Geometry: final body of the model. Coordinates: model frame, mm. A direction names the side the tool comes from. Give positions to 0.01 mm unless a question says otherwise; leave off trailing zeros. Write each loop counter-clockwise with the first axis right and the second up, starting at its lowest first coordinate (ties: lowest second). Pieces come first, ordered by that corner, then holes. Notation, with made-up numbers: M 69.5,69.25 L 115.5,69.25 A15 ccw 115.5,91.25 Z; hole C -29,79.5 d1. An arc over 180 degrees is marked long. Use one line per item in the form item = value. Start each with the question number.
Item 1: Section query C-C on x = 7.75. Return loops of the section in (y, z), then the cut area to 3 significant figures.
Item 2: Material intervals for line 1 along X through (y, z) = (13.5, 200.5); line 2 along Y through (x, z) = (1, 281.5); line 3 along X through (y, z) = (15, 165), sorted ascending. Write a range as from..to.
Item 3: Section query A-A on y = -8. Return loops of the section in (x, z), then the cut area to 3 significant figures.
Item 4: Contact query for a flat-ended pin moving along its axis: P1, Ø3, axis at x = 0.53, z = 190.5, coming from the -Y side. Output: stop coordinate, or through.
Item 5: Pull-direction query (Y, two-part tool) for faces 3 (the flat face through (1, 14.737, 150)), 4 (the flat face through (13.229, -9, 150)), 5 (the flat face through (1, -34.793, 150)); classes: released by +Y, released by -Y, zero draft, split by the parting line, or undercut.
Item 6: Access query for faces 1 (the flat face through (-10.901, -9, 150)), 2 (the flat face through (-12.171, -10, 150)). Directions: +Z, -Z, +X, -X, +Y, -Y. A direction counts if a zero-diameter tool reaches every point of the face in a straight line with its end or side. Return the directions, or none.
Item 7: Section query B-B on z = 108. Return loops of the section in (x, y), then the cut area to 3 significant figures.
Autodesk Inventor part; units mm, degrees
ref_plane "YZ Plane" through (0, 0, 0) normal (1, 0, 0) x (0, 1, 0)
ref_plane "XZ Plane" through (0, 0, 0) normal (0, 1, 0) x (-1, 0, 0)
ref_plane "XY Plane" through (0, 0, 0) normal (0, 0, 1) x (1, 0, 0)
sketch "Sketch1" plane through (0, 0, 0) normal (0, 0, 1) x (1, 0, 0)
  line L0 (-12.1708, 16.0073) -> (13.2292, 16.0073)
  line L1 (13.2292, 16.0073) -> (13.2292, -34.7927)
  line L2 (13.2292, -34.7927) -> (-12.1708, -34.7927)
  line L3 (-12.1708, -34.7927) -> (-12.1708, 16.0073)
  line L4 (11.9592, 14.7373) -> (-10.9008, 14.7373)
  line L5 (-10.9008, 14.7373) -> (-10.9008, -33.5227)
  line L6 (-10.9008, -33.5227) -> (11.9592, -33.5227)
  line L7 (11.9592, -33.5227) -> (11.9592, 14.7373)
  point P0 (0, 0)
  dimension "d0" = 25.4
  dimension "d1" = 50.8
  dimension "d2" = 1.27
extrude "Extrusion1" add sketch "Sketch1" along normal blind 304.8
sketch "Sketch2" plane through (-12.1708, 16.0073, 0) normal (0, 1, 0) x (1, 0, 0)
  circle A0 centre (12.7, -12.7) radius 1.7272
  line L0 (25.4, 0) -> (0, 0)
  line L1 (0, 0) -> (0, -304.8)
  point P0 (12.1708, 0)
  dimension "d5" = 3.4544
  dimension "d6" = 12.7
  dimension "d7" = 12.7
extrude "Extrusion2" cut sketch "Sketch2" against normal through all
pattern_linear "Rectangular Pattern1" count 12 spacing 25.4 along (0, 0, 1) of "Extrusion2"
equation "\"d3\" = d13"
equation "\"d13\" = 304.8"
properties part number "VerseFrame 12in"
Answer sheet:
q1.outline = M -34.79,0 L -33.52,0 L -33.52,304.8 L -34.79,304.8 Z; M 14.74,0 L 16.01,0 L 16.01,304.8 L 14.74,304.8 Z
q1.area = 774 mm2
q2.line_1 = -12.17..-10.9, 11.96..13.23
q2.line_2 = -34.79..-33.52, 14.74..16.01
q2.line_3 = -12.17..-1.2, 2.25..13.23
q3.outline = M -12.17,0 L -10.9,0 L -10.9,304.8 L -12.17,304.8 Z; M 11.96,0 L 13.23,0 L 13.23,304.8 L 11.96,304.8 Z
q3.area = 774 mm2
q4.P1 = through
q5.face_3 = undercut
q5.face_4 = zero draft
q5.face_5 = released by -Y
q6.face_1 = +Z, -Z
q6.face_2 = +Z, -Z, -X, +Y, -Y
q7.outline = M -12.17,-34.79 L 13.23,-34.79 L 13.23,16.01 L -12.17,16.01 Z; hole M -10.9,-33.52 L 11.96,-33.52 L 11.96,14.74 L -10.9,14.74 Z
q7.area = 187 mm2
